```python
from build123d import *

# Parameters (mm, degrees)
F0_W      = 20
F0_H      = 16.9
F0_R      = 1.6
F1_DEPTH  = 10
F2_R      = 2.75
F3_DEPTH  = 5
F4_W      = 35
F4_H      = 45.5
F5_DEPTH  = 10
F6_R      = 3
F7_DEPTH  = 10
F8_R      = 3
F9_DEPTH  = 6.5
F10_R     = 1.75
F11_DEPTH = 10.001
F13_DEPTH = 3.501
F14_R     = 17.6
F15_DEPTH = 3
F16_R     = 3
F17_R     = 5.5
F18_DEPTH = 0.5


with BuildPart() as f1:
    # F0 (on Top) → F1 (new body)
    with BuildSketch(Plane.XY):
        Rectangle(F0_W, F0_H)
        with Locations((-5, 0)):
            Circle(F0_R, mode=Mode.SUBTRACT)
        with Locations((5, 0)):
            Circle(F0_R, mode=Mode.SUBTRACT)
    extrude(amount=-F1_DEPTH)

    # F2 (on face) → F3 (cut)
    with BuildSketch(Plane.XY):
        with Locations((-5, 0)):
            Circle(F2_R)
        with Locations((5, 0)):
            Circle(F2_R)
    extrude(amount=-F3_DEPTH, mode=Mode.SUBTRACT)

    # F4 (on face) → F5 (join)
    with BuildSketch(Plane(origin=(-10, 0, 0), x_dir=(0, -1, 0), z_dir=(-1, 0, 0))):
        with Locations((0, 12.75)):
            Rectangle(F4_W, F4_H)
    extrude(amount=F5_DEPTH)

    # F6 (on face) → F7 (cut, through all)
    with BuildSketch(Plane(origin=(-20, 0, 0), x_dir=(0, -1, 0), z_dir=(-1, 0, 0))):
        with Locations((0, 25)):
            Circle(F6_R)
    extrude(amount=-F7_DEPTH, mode=Mode.SUBTRACT)

    # F8 (on face) → F9 (cut)
    with BuildSketch(Plane.YZ.offset(-10)):
        with BuildLine():
            ThreePointArc((-11.7993208208, 11.9410556258), (0, 14.45), (11.7993208208, 11.9410556258))
            ThreePointArc((11.7993208208, 11.9410556258), (15.6809149912, 17.0081976351), (17.5, 23.1265006005))
            Line((17.5, 23.1265006005), (17.5, 35.5))
            Line((17.5, 35.5), (-17.5, 35.5))
            Line((-17.5, 35.5), (-17.5, 23.1265006005))
            ThreePointArc((-17.5, 23.1265006005), (-15.6809149912, 17.0081976351), (-11.7993208208, 11.9410556258))
        make_face()
        with Locations((0, 25)):
            Circle(F8_R, mode=Mode.SUBTRACT)
    extrude(amount=-F9_DEPTH, mode=Mode.SUBTRACT)

    # F10 (on face) → F11 (cut, through all)
    with BuildSketch(Plane.YZ.offset(-10)):
        with Locations((6, 32.4)):
            Circle(F10_R)
        with Locations((9.5, 17)):
            Circle(F10_R)
        with Locations((-6, 18.5)):
            Circle(F10_R)
        with Locations((-10, 34)):
            Circle(F10_R)
    extrude(amount=-F11_DEPTH, mode=Mode.SUBTRACT)

    # F12 (on face) → F13 (cut, through all)
    with BuildSketch(Plane.YZ.offset(-16.5)):
        Polygon((7.5, 21), (17.5, 21), (17.5, 35.5), (10.4602255331, 35.5), align=None)
    extrude(amount=-F13_DEPTH, mode=Mode.SUBTRACT)

    # F14 (on face) → F15 (cut)
    with BuildSketch(Plane.YZ.offset(-10)):
        with Locations((0, 25)):
            Circle(F14_R)
    extrude(amount=-F15_DEPTH, mode=Mode.SUBTRACT)

    # F16
    f16_edges = [f1.edges().sort_by_distance(p)[0] for p in [
        (-18.25, 10.460226, 35.5),
        (-18.25, -17.5, 35.5),
        (-15, -17.5, -10),
        (-15, 17.5, -10),
    ]]
    fillet(f16_edges, radius=F16_R)

    # F17 (on face) → F18 (cut)
    with BuildSketch(Plane.YZ.offset(-16.5)):
        with Locations((0, 25)):
            Circle(F17_R)
    extrude(amount=-F18_DEPTH, mode=Mode.SUBTRACT)


solid = f1.part
```
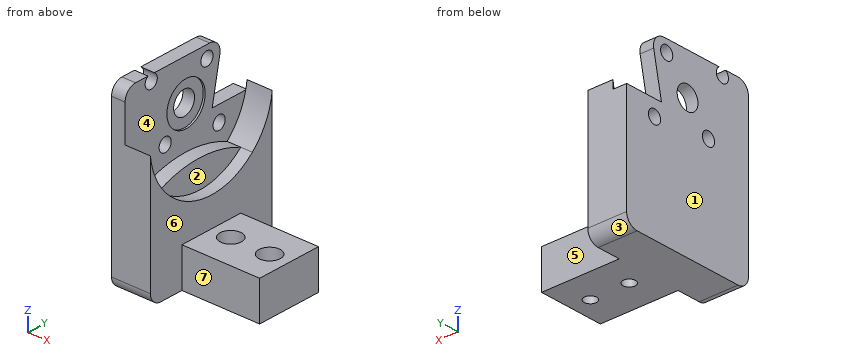
For this review, take the finished solid that the model builds, in its own axes (mm). Face numbers are marked on the shaded views. A direction names the side the tool comes from. Coordinates: 2 decimals unless noted, no trailing zeros. Write each loop counter-clockwise with the first axis right and the second up, starting at its lowest first coordinate (ties: lowest second). Pieces come first, ordered by that corner, then holes.
(1) Add section C-C on y = -1. Count the separate pieces of the cut face and the enclosed holes in it, then the cut area to 3 significant figures.
(2) Tool access review of the marked faces 5, 6 and 7: name each direction out of +Z, -Z, +X, -X, +Y, -Y from which nothing blocks a thin tool from reaching the whole face with its end or side.
(3) Add section B-B on x = -15.5. Give the boundary of the cut face in (y, z), then the cut area to 3 significant figures.
(4) Wall thickness on probe 1 along Y at (x, z) = (-5, -4); probe 2 along Y at (x, z) = (-5, -6.65); probe 3 along Z at (x, y) = (-18.9, 0): over which ranges is each line inside the solid? List them lowest first.
(5) The part is to be moulded in two halves that separate along Y. For the marked faces 1, 2, 3 and 4, say which applies: +Y half, -Y half, draft (parallel to the pull), parting line (faces both ways), or undercut.
(6) Add section A-A on z = -2.5. Give the boundary of the cut face in (x, y).
(7) For pin 1 Ø3.5 at (x, y) = (-5, 0) entering from +Z; pin 2 Ø1.8 at (x, y) = (-18, 11.5) entering from +Z; pin 3 Ø8.5 at (x, y) = (-0.5, 2) entering from +Z; pin 4 Ø3 at (y, z) = (6, 32.4) entering from +X, all flat-tipped, find the tip position at first contact; note any pin that passes through.
(8) Add section D-D on y = -10. Give the boundary of the cut face in (x, z), then the cut area to 3 significant figures.
Answer sheet:
1. separate pieces: 4
1. enclosed holes: 0
1. area: 398 mm2
2. face 5: +Z, -Z, +X, +Y
2. face 6: +Z, +X
2. face 7: +Z, -Z, +X, -Y
3. outline: (-17.5, -7) arc R3 ccw to (-14.5, -10) - (14.5, -10) arc R3 ccw to (17.5, -7) - (17.5, 23.13) arc R17.6 cw to (11.8, 11.94) arc R29 ccw to (-11.8, 11.94) arc R17.6 cw to (-17.5, 23.13) - close
3. area: 848 mm2
4. probe 1: y = -8.45 to -2.75, 2.75 to 8.45
4. probe 2: y = -8.45 to -1.6, 1.6 to 8.45
4. probe 3: z = -10 to 22, 28 to 35.5
5. face 1: draft
5. face 2: undercut
5. face 3: +Y half
5. face 4: undercut
6. outline: (-20, -17.5) - (-10, -17.5) - (-10, -8.45) - (10, -8.45) - (10, 8.45) - (-10, 8.45) - (-10, 17.5) - (-20, 17.5) - close; hole circle Ø5.5 at (-5, 0); hole circle Ø5.5 at (5, 0)
7. pin 1: stops at z = -5
7. pin 2: stops at z = 21
7. pin 3: stops at z = 0
7. pin 4: passes through
8. outline: (-20, -10) - (-10, -10) - (-10, 10.52) - (-13, 10.52) - (-13, 12.67) - (-16.5, 12.67) - (-16.5, 32.25) - (-20, 32.25) - close
8. area: 289 mm2
